from build123d import *

# Parameters (mm, degrees)
CROQUIS1_W              = 4.765
CROQUIS1_H              = 20
SALIENTE_EXTRUIR1_DEPTH = 2.5


with BuildPart() as part:
    # Croquis1 → Revolución1 (revolve)
    with BuildSketch(Plane.XY):
        with Locations((2.3825, 10)):
            Rectangle(CROQUIS1_W, CROQUIS1_H)
    revolve(axis=Axis((0, 0, 0), (0, 1, 0)))

    # Croquis2 → Saliente-Extruir1 (add)
    with BuildSketch(Plane(origin=(0, 20, 0), x_dir=(1, 0, 0), z_dir=(0, 1, 0))):
        Polygon((-7.332348419, 0), (-3.666174209, -6.35), (3.666174209, -6.35), (7.332348419, 0), (3.666174209, 6.35), (-3.666174209, 6.35), align=None)
    extrude(amount=SALIENTE_EXTRUIR1_DEPTH)


solid = part.part
Model file for the job. Use its own axes, mm. A direction names the side the tool comes from. Give positions to 0.01 mm unless a question says otherwise; leave off trailing zeros. Loops run counter-clockwise (first coordinate to the right, second up) from the corner with the lowest first, then second, coordinate; pieces in that order, holes last. Notation, with made-up numbers: (-18, -18.5) -> (6, -18.5) arc R27 ccw to (6, 4.5) -> close; hole circle Ø4 at (29, -37.5). An arc over 180 degrees is marked (long way). Use a Markdown table: item, result. Add a question column.
(1) Drop flat-ended pins along their axis: pin 1 Ø3 at (x, y) = (-3, 7) entering from -Z; pin 2 Ø8 at (x, y) = (-4.5, 4) entering from -Z; pin 3 Ø5 at (x, y) = (-0.5, 12.5) entering from +Z (3 decimals). Give the stop position or say it passes through.
(2) Slice it at D-D on x = -5.5. List the corners of the cut face in (y, z).
(3) Slice it at B-B on z = 4. List the corners of the cut face in (x, y).
(4) Wall check: line 1 along Y through (x, z) = (-6, 2.25); line 2 along X through (y, z) = (13.5, -3.75); line 3 along Z through (x, y) = (2.25, 15.75). Give the ranges that are in metal, low to high.
(5) Slice it at C-C on y = 7. List the corners of the cut face in (x, z) (3 decimals).
(6) Tool access for faces 1 (the flat face through (5.474, 21.232, 3.219)), 2 (the cylindrical face through (-0.62, 10.14, -4.724)): list every direction of +Z, -Z, +X, -X, +Y, -Y with a clear straight run to the whole face (end or side of a thin tool).
(7) Slice it at A-A on x = 0. List the corners of the cut face in (y, z) (3 decimals), and give its area (3 significant figures).
(8) Mould opens along Z. For faces 3 (the flat face through (-5.525, 21.232, 3.131)), 4 (the flat face through (5.525, 21.232, -3.131)), 5 (the flat face through (0, 22.5, 0)) say: +Z half, -Z half, draft (parallel to the pull), parting line (faces both ways), or undercut.
Filled sheet:
| question | item | result |
|---|---|---|
| 1 | pin 1 | z = -4.52 |
| 1 | pin 2 | z = -4.74 |
| 1 | pin 3 | z = 4.765 |
| 2 | outline | (20, -3.17) -> (22.5, -3.17) -> (22.5, 3.17) -> (20, 3.17) -> close |
| 3 | outline | (-5.02, 20) -> (-2.59, 20) -> (-2.59, 0) -> (2.59, 0) -> (2.59, 20) -> (5.02, 20) -> (5.02, 22.5) -> (-5.02, 22.5) -> close |
| 4 | line 1 | 20 to 22.5 |
| 4 | line 2 | -2.94 to 2.94 |
| 4 | line 3 | -4.2 to 4.2 |
| 5 | outline | circle Ø9.53 at (0, 0) |
| 6 | face 1 | +Z, +X, +Y, -Y |
| 6 | face 2 | -Y |
| 7 | outline | (0, -4.765) -> (20, -4.765) -> (20, -6.35) -> (22.5, -6.35) -> (22.5, 6.35) -> (20, 6.35) -> (20, 4.765) -> (0, 4.765) -> close |
| 7 | area | 222 mm2 |
| 8 | face 3 | +Z half |
| 8 | face 4 | -Z half |
| 8 | face 5 | draft |
